Build history of the part. All positions in model axes, mm. Round coordinates to 2 decimals unless told otherwise and drop trailing zeros. Loops run counter-clockwise (first coordinate to the right, second up) from the corner with the lowest first, then second, coordinate; pieces in that order, holes last.
from build123d import *

# Parameters (mm, degrees)
SKETCH_R    = 5
PAD_DEPTH   = 100
SKETCH001_R = 2.1
HOLE_DEPTH  = 600.999753


with BuildPart() as part:
    # Sketch → Pad (new body, symmetric)
    with BuildSketch(Plane.XY):
        Circle(SKETCH_R)
    extrude(amount=PAD_DEPTH, both=True)

    # Sketch001 (on Face3 of Pad) → Hole (cut, through all)
    with BuildSketch(Plane.XY.offset(100)):
        Circle(SKETCH001_R)
    hole = extrude(amount=-HOLE_DEPTH, mode=Mode.SUBTRACT)

    # Mirrored: Hole across XY
    add(hole.mirror(Plane.XY), mode=Mode.SUBTRACT)


solid = part.part
(1) Slice it at A-A on x = 0. List the corners of the cut face in (y, z).
Responses:
outline: (-5, -100) - (-2.1, -100) - (-2.1, 100) - (-5, 100) - close; (2.1, -100) - (5, -100) - (5, 100) - (2.1, 100) - close
(2) Probe line 1 (Y direction, x = 0, z = -25.5); line 2 (X direction, y = -0.75, z = 11); line 3 (X direction, y = -0.5, z = 73). List the from-to ranges inside material, lowest first.
Responses:
line 1: y = -5 to -2.1, 2.1 to 5
line 2: x = -4.94 to -1.96, 1.96 to 4.94
line 3: x = -4.97 to -2.04, 2.04 to 4.97
(3) Pin check, flat tip, straight feed: P1, Ø5, axis at y = -3, z = -22, coming from the +X side. Stop position of the tip, or through.
Responses:
P1: stops at x = 4.97
(4) Pull direction X, two halves, no side cores. Call faces 1 (the face through (-1.08, -4.88, 1.4)), 2 (the face through (2.003, 0.631, 1.4)), 3 (the face through (1, -2.2, -100)): +X half, -X half, draft (parallel to the pull), parting line (faces both ways), or undercut.
Responses:
face 1: parting line
face 2: undercut
face 3: draft
(5) Slice it at C-C on z = 21.5. List the corners of the cut face in (x, y).
Responses:
outline: circle Ø10 at (0, 0); hole circle Ø4.2 at (0, 0)
